from build123d import *

# Parameters (mm, degrees)
SKETCH_R           = 11
PAD_DEPTH          = 2
SKETCH001_R        = 5
PAD001_DEPTH       = 10
SKETCH002_R        = 2.5
POCKET_DEPTH       = 12.001
SKETCH003_R        = 1.55
POCKET001_DEPTH    = 78.694328
POLARPATTERN_COUNT = 4
FILLET_R           = 0.4


with BuildPart() as part:
    # Sketch → Pad (new body)
    with BuildSketch(Plane.XY):
        Circle(SKETCH_R)
    extrude(amount=PAD_DEPTH)

    # Sketch001 (on Face3 of Pad) → Pad001 (join)
    with BuildSketch(Plane.XY.offset(2)):
        Circle(SKETCH001_R)
    extrude(amount=PAD001_DEPTH)

    # Sketch002 (on Face5 of Pad001) → Pocket (cut, through all)
    with BuildSketch(Plane.XY.offset(12)):
        Circle(SKETCH002_R)
    extrude(amount=-POCKET_DEPTH, mode=Mode.SUBTRACT)

    # Sketch003 (on Face2 of Pocket) → Pocket001 (cut, through all)
    with BuildSketch(Plane(origin=(0, 0, 0), x_dir=(1, 0, 0), z_dir=(0, 0, -1))):
        with Locations((0, 7.5)):
            Circle(SKETCH003_R)
    pocket001 = extrude(amount=-POCKET001_DEPTH, mode=Mode.SUBTRACT)

    # PolarPattern: Pocket001 ×4 about axis
    polarpattern_axis = Axis((0, 0, 0), (0, 0, -1))
    for i in range(1, POLARPATTERN_COUNT):
        add(pocket001.rotate(polarpattern_axis, i * 360 / POLARPATTERN_COUNT), mode=Mode.SUBTRACT)

    # Fillet
    fillet_edges = [part.edges().sort_by_distance(p)[0] for p in [
        (-5, 0, 12),
        (-7.5, -1.55, 1),
        (-11, 0, 2),
        (-11, 0, 0),
        (-7.5, 1.55, 0),
    ]]
    fillet(fillet_edges, radius=FILLET_R)


solid = part.part
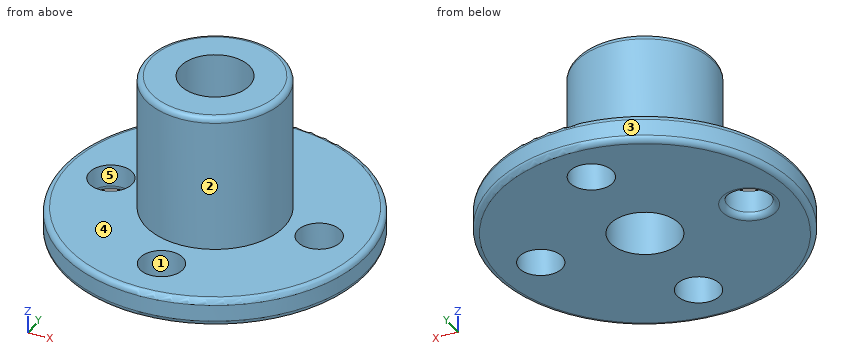
The listing builds one solid part. Answer for the finished solid, in the listing's coordinates (mm). Face numbers are marked on the shaded views. A direction names the side the tool comes from. Give positions to 0.01 mm unless a question says otherwise; leave off trailing zeros. Write each loop counter-clockwise with the first axis right and the second up, starting at its lowest first coordinate (ties: lowest second). Pieces come first, ordered by that corner, then holes. Notation, with made-up numbers: (87.5, 20) -> (136.5, 20) arc R14 cw to (136.5, 42) -> close; hole circle Ø5 at (-8.75, -7). An arc over 180 degrees is marked (long way). One line per question, with ' | ' between items. Start each with the question number.
1. Section B-B (x = 0) is taken. Determine the outline of the cut face in (y, z), plus the area to 3 significant figures.
2. Section C-C (z = 5.25) is taken. Determine the outline of the cut face in (x, y).
3. Find the intervals of material crossed by probe 1 along Y at (x, z) = (0, 0.55); probe 2 along Y at (x, z) = (0, 4.25); probe 3 along Z at (x, y) = (-3.25, -8), in increasing order.
4. Section A-A (y = 0) is taken. Determine the outline of the cut face in (x, z).
5. For a pull along X with two mould halves and no side action, classify the marked faces 3, 4 and 5 as pulls with the +X half, pulls with the -X half, needs draft (parallel to the pull), parting line crosses it, or undercut.
6. Given pin 1 Ø12 at (x, y) = (6.5, 7) entering from +Z; pin 2 Ø4 at (x, z) = (-3.5, 2) entering from -Y; pin 3 Ø2 at (y, z) = (3, 8.5) entering from +X; pin 4 Ø3 at (x, z) = (-1, 8) entering from +Y, each flat-ended and moving along its own axis, determine where each tip first touches the part or whether it passes through.
7. For the marked faces 1 and 2, determine the directions among +Z, -Z, +X, -X, +Y, -Y from which every point of the face is accessible in a straight line to the end or side of a thin tool.
Response values:
1) outline: (-11, 0.4) arc R0.4 ccw to (-10.6, 0) -> (-9.05, 0) -> (-9.05, 2) -> (-10.6, 2) arc R0.4 ccw to (-11, 1.6) -> close; (-5.95, 0) -> (-2.5, 0) -> (-2.5, 12) -> (-4.6, 12) arc R0.4 ccw to (-5, 11.6) -> (-5, 2) -> (-5.95, 2) -> close; (2.5, 0) -> (5.95, 0) -> (5.95, 2) -> (5, 2) -> (5, 11.6) arc R0.4 ccw to (4.6, 12) -> (2.5, 12) -> close; (9.05, 0) -> (10.6, 0) arc R0.4 ccw to (11, 0.4) -> (11, 1.6) arc R0.4 ccw to (10.6, 2) -> (9.05, 2) -> close | area: 71.4 mm2
2) outline: circle Ø10 at (0, 0); hole circle Ø5 at (0, 0)
3) probe 1: -11 to -9.05, -5.95 to -2.5, 2.5 to 5.95, 9.05 to 11 | probe 2: -5 to -2.5, 2.5 to 5 | probe 3: 0 to 2
4) outline: (-11, 0.4) arc R0.4 ccw to (-10.6, 0) -> (-9.45, 0) arc R0.4 ccw to (-9.05, 0.4) -> (-9.05, 2) -> (-10.6, 2) arc R0.4 ccw to (-11, 1.6) -> close; (-5.95, 0.4) arc R0.4 ccw to (-5.55, 0) -> (-2.5, 0) -> (-2.5, 12) -> (-4.6, 12) arc R0.4 ccw to (-5, 11.6) -> (-5, 2) -> (-5.95, 2) -> close; (2.5, 0) -> (5.95, 0) -> (5.95, 2) -> (5, 2) -> (5, 11.6) arc R0.4 ccw to (4.6, 12) -> (2.5, 12) -> close; (9.05, 0) -> (10.6, 0) arc R0.4 ccw to (11, 0.4) -> (11, 1.6) arc R0.4 ccw to (10.6, 2) -> (9.05, 2) -> close
5) face 3: parting line crosses it | face 4: needs draft | face 5: undercut
6) pin 1: z = 12 | pin 2: y = -10.89 | pin 3: x = 4.58 | pin 4: y = 5
7) face 1: +Z, -Z | face 2: +Z
